Check sheet for the modelled part. Datum: model origin and axes. Units: mm. A direction names the side the tool comes from. Give positions to 0.01 mm unless a question says otherwise; leave off trailing zeros. Order: outer loops, then holes, each group sorted by start corner. A loop starts at its lowest first (then second) coordinate and runs counter-clockwise, first axis right, second up. Notation, with made-up numbers: (-23.75, -18) -> (-18.75, -18) arc R24 cw to (-18.75, 16) -> close; hole circle Ø10 at (17.25, 47.25). An arc over 180 degrees is marked (long way). One line per question, with ' | ' between items. Start each with the question number.
from build123d import *

# Parameters (mm, degrees)
SKETCH1_W               = 6.35
SKETCH1_H               = 16.51
SKETCH1_R               = 1.905
BOSS_EXTRUDE1_DEPTH     = 7.62
SKETCH2_W               = 6.35
SKETCH2_H               = 2.794
CUT_EXTRUDE1_DEPTH      = 1
CUT_EXTRUDE1_DEPTH_BACK = 8.89
SKETCH4_R               = 1.8415
CUT_EXTRUDE2_DEPTH      = 7.35


with BuildPart() as part:
    # Sketch1 → Boss-Extrude1 (new body)
    with BuildSketch(Plane(origin=(0, 0, 0), x_dir=(1, 0, 0), z_dir=(0, 1, 0))):
        with Locations((3.175, 8.255)):
            Rectangle(SKETCH1_W, SKETCH1_H)
        with Locations((3.175, 3.175)):
            Circle(SKETCH1_R, mode=Mode.SUBTRACT)
    extrude(amount=BOSS_EXTRUDE1_DEPTH)

    # Sketch2 → Cut-Extrude1 (cut, two sides)
    with BuildSketch(Plane.XY) as cut_extrude1_sk:
        with Locations((3.175, 3.81)):
            Rectangle(SKETCH2_W, SKETCH2_H)
    extrude(amount=CUT_EXTRUDE1_DEPTH, mode=Mode.SUBTRACT)
    extrude(cut_extrude1_sk.sketch, amount=-CUT_EXTRUDE1_DEPTH_BACK, mode=Mode.SUBTRACT)

    # Sketch4 → Cut-Extrude2 (cut, through all)
    with BuildSketch(Plane(origin=(6.35, 0, 0), x_dir=(0, 0, -1), z_dir=(1, 0, 0))):
        with Locations((12.827, 3.81)):
            Circle(SKETCH4_R)
    extrude(amount=-CUT_EXTRUDE2_DEPTH, mode=Mode.SUBTRACT)


solid = part.part
1. Cross-section at D-D on y = 1.25. Record the boundary of the cut face in (x, z) (3 decimals).
2. Tool access check on faces 1 (the face through (3.1, 2.413, -5.4)), 2 (the face through (3, 4, -16.51)). Record the directions out of +Z, -Z, +X, -X, +Y, -Y that give a thin tool (end or side, any length) a straight path to the whole face; none if there is none.
3. Cross-section at B-B on y = 3.81. Record the boundary of the cut face in (x, z).
4. Cross-section at C-C on x = 2. Record the boundary of the cut face in (y, z), and give its area (3 significant figures).
5. Mould release check, pull along Z, two halves, no side actions. Record for faces 3 (the face through (3, 0, -8)), 4 (the face through (3, 1, 0)), 5 (the face through (3.219, 3.891, -10.987)), 6 (the face through (2.927, 6.397, -5.064)): +Z half, -Z half, draft (parallel to the pull), parting line (faces both ways), or undercut.
6. Scan lines: probe 1 along Y at (x, z) = (5.25, -1.5); probe 2 along Z at (x, y) = (3.25, 1.5); probe 3 along Z at (x, y) = (3.25, 3). Record each from-to range of solid material in increasing order.
7. Go/stop test with a flat-tipped pin: pin 1 (0.8 mm diameter, centred on x = 3.5, y = 4, fed in from +Z). Record where the tip stops, or that it passes through.
8. Cross-section at A-A on z = -1. Record the boundary of the cut face in (x, y), and give its area (3 significant figures).
Response values:
1) outline: (0, -16.51) -> (6.35, -16.51) -> (6.35, 0) -> (0, 0) -> close; hole circle Ø3.81 at (3.175, -3.175)
2) face 1: +Z, +X, -X | face 2: -Z, +X, -X, +Y, -Y
3) outline: (0, -16.51) -> (6.35, -16.51) -> (6.35, -14.67) -> (0, -14.67) -> close; (0, -10.99) -> (6.35, -10.99) -> (6.35, -8.89) -> (0, -8.89) -> close
4) outline: (0, -16.51) -> (7.62, -16.51) -> (7.62, -4.67) -> (5.21, -4.67) -> (5.21, -8.89) -> (2.41, -8.89) -> (2.41, -4.67) -> (0, -4.67) -> close; (0, -1.68) -> (2.41, -1.68) -> (2.41, 0) -> (0, 0) -> close; (5.21, -1.68) -> (7.62, -1.68) -> (7.62, 0) -> (5.21, 0) -> close; hole circle Ø3.68 at (3.81, -12.83) | area: 75.8 mm²
5) face 3: draft | face 4: +Z half | face 5: undercut | face 6: undercut
6) probe 1: y = 0 to 2.41, 5.21 to 7.62 | probe 2: z = -16.51 to -5.08, -1.27 to 0 | probe 3: z = -16.51 to -14.48, -11.17 to -8.89
7) pin 1: stops at z = -8.89
8) outline: (0, 0) -> (6.35, 0) -> (6.35, 2.41) -> (0, 2.41) -> close; (0, 5.21) -> (6.35, 5.21) -> (6.35, 7.62) -> (0, 7.62) -> close | area: 30.6 mm²
